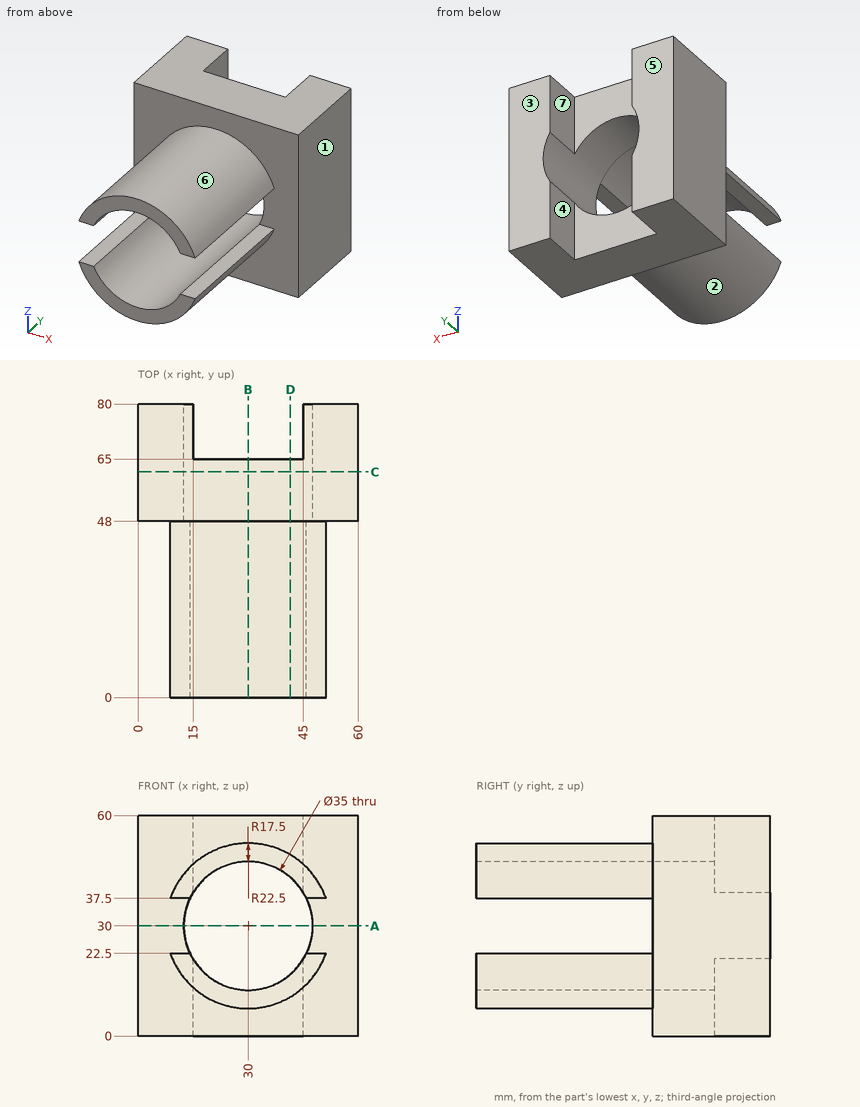
Geometry: see drawing. Coordinates: mm, zero at the bounding-box minimum. A direction names the side the tool comes from. Round coordinates to 2 decimals unless told otherwise and drop trailing zeros. Loops run counter-clockwise (first coordinate to the right, second up) from the corner with the lowest first, then second, coordinate; pieces in that order, holes last. Notation, with made-up numbers: (-12, 57.25) -> (14, 57.25) arc R15 ccw to (14, 79.25) -> close; hole circle Ø6 at (81, -18). An arc over 180 degrees is marked (long way). Use one line per item in the form item = value. Start each with the question number.
Item 1: Mould query, pull axis X, two halves, no side actions, for the marked faces 1, 2, 3 and 4. Classes: pulls with the +X half, pulls with the -X half, needs draft (parallel to the pull), parting line crosses it, or undercut.
Item 2: Material intervals for L1, parallel to Z at x = 30, y = 50; L2, parallel to Y at x = 27.5, z = 10.5, sorted ascending. Write a range as from..to.
Item 3: Section query D-D on x = 41.5. Return the cut outline in (y, z), then the cut area to 3 significant figures.
Item 4: Set-up query: the marked faces 5, 6 and 7. Return all of +Z, -Z, +X, -X, +Y, -Y with unobstructed straight access to the full face (end or side cutting, diameter ignored); none if empty.
Item 5: Section query A-A on z = 30. Return the cut outline in (x, y).
Item 6: Section query C-C on y = 61.5. Return the cut outline in (x, z).
Item 7: Section query B-B on x = 30. Return the cut outline in (y, z).
Item 8: Contact query for flat-ended pins moving along their axis: pin 1 Ø3 at (y, z) = (38, 41.5) entering from +X; pin 2 Ø12 at (y, z) = (73.5, 9.5) entering from -X; pin 3 Ø4.5 at (x, y) = (12, 33) entering from +Z; pin 4 Ø4.5 at (x, y) = (47.5, 18) entering from -Z. Output: stop coordinate, or through.
Ans:
q1.face_1 = pulls with the +X half
q1.face_2 = parting line crosses it
q1.face_3 = needs draft
q1.face_4 = undercut
q2.L1 = 0..12.5, 47.5..60
q2.L2 = 0..65
q3.outline = (0, 10.66) -> (48, 10.66) -> (48, 0) -> (65, 0) -> (65, 16.81) -> (0, 16.81) -> close; (0, 43.19) -> (65, 43.19) -> (65, 60) -> (48, 60) -> (48, 49.34) -> (0, 49.34) -> close
q3.area = 1,160 mm^2
q4.face_5 = +Z, -Z, +X, -X, +Y
q4.face_6 = +Z, -Y
q4.face_7 = +Z, -Z, +Y
q5.outline = (0, 48) -> (12.5, 48) -> (12.5, 80) -> (0, 80) -> close; (47.5, 48) -> (60, 48) -> (60, 80) -> (47.5, 80) -> close
q6.outline = (0, 0) -> (60, 0) -> (60, 60) -> (0, 60) -> close; hole circle Ø35 at (30, 30)
q7.outline = (0, 7.5) -> (48, 7.5) -> (48, 0) -> (65, 0) -> (65, 12.5) -> (0, 12.5) -> close; (0, 47.5) -> (65, 47.5) -> (65, 60) -> (48, 60) -> (48, 52.5) -> (0, 52.5) -> close
q8.pin_1 = 50.16
q8.pin_2 = 0
q8.pin_3 = 46.07
q8.pin_4 = 13.46
